```python
from build123d import *

# Parameters (mm, degrees)
DODANIE_WYCI_GNI_CIE1_DEPTH = 50
SZKIC2_R                    = 4.25
WYTNIJ_WYCI_GNI_CIE1_DEPTH  = 21
SFAZOWANIE1_START           = -60.634406487
SFAZOWANIE1_OUTLINE_W       = 4.242640687
SFAZOWANIE1_OUTLINE_H       = 50
SFAZOWANIE1_DEPTH           = 2.634406487
SFAZOWANIE2_START           = 58
SFAZOWANIE2_OUTLINE_W       = 4.242640687
SFAZOWANIE2_OUTLINE_H       = 50
SFAZOWANIE2_DEPTH           = 2.634406487


with BuildPart() as part:
    # Szkic1 → Dodanie-wyci_gni_cie1 (new body)
    with BuildSketch(Plane.XY):
        with BuildLine():
            Line((70.75, 0), (100.75, 0))
            Line((100.75, 0), (100.75, -5))
            Line((100.75, -5), (77.75, -5))
            Line((77.75, -5), (77.75, -78.737292332))
            Line((77.75, -78.737292332), (38.85, -78.737292332))
            Line((38.85, -78.737292332), (38.85, -98.737292332))
            Line((38.85, -98.737292332), (25, -98.737292332))
            Line((25, -98.737292332), (25, -78.737292332))
            Line((25, -78.737292332), (-25, -78.737292332))
            Line((-25, -78.737292332), (-25, -98.737292332))
            Line((-25, -98.737292332), (-38.85, -98.737292332))
            Line((-38.85, -98.737292332), (-38.85, -78.737292332))
            Line((-38.85, -78.737292332), (-77.75, -78.737292332))
            Line((-77.75, -78.737292332), (-77.75, -5))
            Line((-77.75, -5), (-100.75, -5))
            Line((-100.75, -5), (-100.75, 0))
            Line((-100.75, 0), (-70.75, 0))
            ThreePointArc((-70.75, 0), (0, -70.75), (70.75, 0))
        make_face()
    extrude(amount=DODANIE_WYCI_GNI_CIE1_DEPTH)

    # Szkic2 → Wytnij-wyci_gni_cie1 (cut)
    with BuildSketch(Plane(origin=(0, 0, 0), x_dir=(1, 0, 0), z_dir=(0, 1, 0))):
        with Locations(Location((-90.75, -10, 0), (0, 0, 270))):
            Circle(SZKIC2_R)
        with Locations(Location((-90.75, -40, 0), (0, 0, 270))):
            Circle(SZKIC2_R)
    wytnij_wyci_gni_cie1 = extrude(amount=-WYTNIJ_WYCI_GNI_CIE1_DEPTH, mode=Mode.SUBTRACT)

    # Lustro2: Wytnij-wyci_gni_cie1 across plane
    add(wytnij_wyci_gni_cie1.mirror(Plane(origin=(0, 0, 0), x_dir=(0, 0, 1), z_dir=(1, 0, 0))), mode=Mode.SUBTRACT)

    # Sfazowanie1: read off the stored shape, not the designer's step
    # Sfazowanie1 outline → Sfazowanie1 (add)
    with BuildSketch(Plane(origin=(0, 0, 0), x_dir=(0.707106781186548, -0.707106781186547, 0), z_dir=(0.707106781186547, 0.707106781186548, 0)).offset(SFAZOWANIE1_START)):
        with Locations((-51.442018332, -25)):
            Rectangle(SFAZOWANIE1_OUTLINE_W, SFAZOWANIE1_OUTLINE_H)
    extrude(amount=SFAZOWANIE1_DEPTH)

    # Sfazowanie2: read off the stored shape, not the designer's step
    # Sfazowanie2 outline → Sfazowanie2 (add)
    with BuildSketch(Plane(origin=(0, 0, 0), x_dir=(0.7071067811865471, 0.707106781186548, 0), z_dir=(0.707106781186548, -0.707106781186547, 0)).offset(SFAZOWANIE2_START)):
        with Locations((51.442018332, 25)):
            Rectangle(SFAZOWANIE2_OUTLINE_W, SFAZOWANIE2_OUTLINE_H)
    sfazowanie2 = extrude(amount=SFAZOWANIE2_DEPTH)

    # Lustro1: Sfazowanie2 across plane
    add(sfazowanie2.mirror(Plane(origin=(0, 0, 0), x_dir=(0, 0, 1), z_dir=(1, 0, 0))))


solid = part.part
```
The model under review builds one solid part; all positions refer to its coordinate system, in mm. A direction names the side the tool comes from. Coordinates: 2 decimals unless noted, no trailing zeros. Write each loop counter-clockwise with the first axis right and the second up, starting at its lowest first coordinate (ties: lowest second). Pieces come first, ordered by that corner, then holes. Notation, with made-up numbers: (53, 45) - (90, 45) arc R15 ccw to (90, 60) - close; hole circle Ø2 at (11, 88). An arc over 180 degrees is marked (long way). Answer in a Markdown table with one row per item. Add a question column.
Q1. Draft analysis for pull direction X (two halves, no side actions). For faces 1 (the face through (-100.75, -3, 25)), 2 (the face through (-25, -89, 25)), 3 (the face through (38.85, -89, 25)), state which applies: +X half, -X half, draft (parallel to the pull), parting line (faces both ways), or undercut.
Q2. To check wall thickness, follow line 1 along Z through (x, y) = (90.75, -1.8); line 2 along X through (y, z) = (-1.55, 40); line 3 along X through (y, z) = (-32, 37). State the ranges of each line that lie inside material, in increasing order. Write a range as from..to.
Q3. Consider section C-C on x = 90.75. Give the boundary of the cut face in (y, z).
Q4. Consider section A-A on z = 40. Give the boundary of the cut face in (x, y).
Q5. Consider section D-D on z = 22.5. Give the boundary of the cut face in (x, y), then the cut area to 3 significant figures.
Q6. For faces 4 (the face through (0, -78.737, 25)), 5 (the face through (91, -5, 25)), 6 (the face through (93.3, -2.5, 36.6)), 7 (the face through (-91, -5, 25)), 8 (the face through (0, -71, 0)), list the 3-axis set-ups (+Z, -Z, +X, -X, +Y, -Y) from which the entire face can be reached by the end or side of a thin tool; tool diameter is ignored.
Q7. Clearance check with flat-ended pins moving along their axes: pin 1 (19.5 mm diameter, centred on x = -56, z = 33, fed in from -Y); pin 2 (12 mm diameter, centred on x = -23.5, z = 8, fed in from +Y); pin 3 (10 mm diameter, centred on x = 90.75, z = 10, fed in from -Y). State where each tip first meets the part, or that it passes through.
Q8. Consider section B-B on y = -60.5. Give the boundary of the cut face in (x, z).
Answers below:
| question | item | result |
|---|---|---|
| 1 | face 1 | -X half |
| 1 | face 2 | undercut |
| 1 | face 3 | +X half |
| 2 | line 1 | 0..5.75, 14.25..35.75, 44.25..50 |
| 2 | line 2 | -100.75..-95, -86.5..-70.73, 70.73..86.5, 95..100.75 |
| 2 | line 3 | -77.75..-63.1, 63.1..77.75 |
| 3 | outline | (-5, 0) - (0, 0) - (0, 5.75) - (-5, 5.75) - close; (-5, 14.25) - (0, 14.25) - (0, 35.75) - (-5, 35.75) - close; (-5, 44.25) - (0, 44.25) - (0, 50) - (-5, 50) - close |
| 4 | outline | (-100.75, -5) - (-95, -5) - (-95, 0) - (-100.75, 0) - close; (-86.5, -5) - (-80.75, -5) - (-77.75, -8) - (-77.75, -78.74) - (-38.85, -78.74) - (-38.85, -98.74) - (-25, -98.74) - (-25, -78.74) - (25, -78.74) - (25, -98.74) - (38.85, -98.74) - (38.85, -78.74) - (77.75, -78.74) - (77.75, -8) - (80.75, -5) - (86.5, -5) - (86.5, 0) - (70.75, 0) arc R70.75 cw to (-70.75, 0) - (-86.5, 0) - close; (95, -5) - (100.75, -5) - (100.75, 0) - (95, 0) - close |
| 5 | outline | (-100.75, -5) - (-80.75, -5) - (-77.75, -8) - (-77.75, -78.74) - (-38.85, -78.74) - (-38.85, -98.74) - (-25, -98.74) - (-25, -78.74) - (25, -78.74) - (25, -98.74) - (38.85, -98.74) - (38.85, -78.74) - (77.75, -78.74) - (77.75, -8) - (80.75, -5) - (100.75, -5) - (100.75, 0) - (70.75, 0) arc R70.75 cw to (-70.75, 0) - (-100.75, 0) - close |
| 5 | area | 5,170 mm² |
| 6 | face 4 | +Z, -Z, -Y |
| 6 | face 5 | +Z, -Z, +X, -Y |
| 6 | face 6 | +Y, -Y |
| 6 | face 7 | +Z, -Z, -X, -Y |
| 6 | face 8 | -Z, +X, -X, +Y, -Y |
| 7 | pin 1 | y = -78.74 |
| 7 | pin 2 | y = -64.31 |
| 7 | pin 3 | y = -5 |
| 8 | outline | (-77.75, 0) - (-36.68, 0) - (-36.68, 50) - (-77.75, 50) - close; (36.68, 0) - (77.75, 0) - (77.75, 50) - (36.68, 50) - close |
